Autodesk Inventor part; units mm, degrees
ref_plane "YZ Plane" through (0, 0, 0) normal (1, 0, 0) x (0, 1, 0)
ref_plane "XZ Plane" through (0, 0, 0) normal (0, 1, 0) x (-1, 0, 0)
ref_plane "XY Plane" through (0, 0, 0) normal (0, 0, 1) x (1, 0, 0)
sketch "Sketch1" plane through (0, 0, 0) normal (1, 0, 0) x (0, 1, 0)
  line L0 (15.4505, 45.3153) -> (5.4505, 45.3153)
  line L1 (5.4505, 45.3153) -> (5.4505, 35.3153)
  line L2 (5.4505, 35.3153) -> (15.4505, 35.3153)
  line L3 (15.4505, 35.3153) -> (15.4505, 45.3153)
  line L4 (29.1713, -4.6847) -> (-18.7008, -4.6847)
  point P0 (0, 0)
  dimension "d0" = 10
  dimension "d1" = 10
  dimension "d3" = 100
revolve "Revolution1" add sketch "Sketch1" angle 360 about axis through (0, 29.1713, -4.6847) along (0, -1, 0)
chamfer "Chamfer1" distance 1 angle 45 4 edges at (0, 15.4505, -54.6847) (0, 5.4505, -54.6847) (0, 15.4505, -44.6847) (0, 5.4505, -44.6847)
properties part number "bearing100-80-10" material "Steel, Galvanized"
Geometry check sheet. Reference: the model listing, model coordinates, mm. Round coordinates to 2 decimals unless told otherwise and drop trailing zeros. Write each loop counter-clockwise with the first axis right and the second up, starting at its lowest first coordinate (ties: lowest second). Pieces come first, ordered by that corner, then holes. Notation, with made-up numbers: (86, -38.75) - (113, -38.75) arc R18 cw to (113, -15.75) - close; hole circle Ø6 at (89.25, 20). An arc over 180 degrees is marked (long way). Write each question's results on one line, items separated by ' | '.
(1) Depth check by flat-ended pin: pin 1 Ø1 at (x, z) = (37, -19.5) entering from -Y; pin 2 Ø4 at (x, y) = (12.5, 8.5) entering from -Z; pin 3 Ø2 at (y, z) = (8, -32.5) entering from +X. Enter the tip coordinate at first touch or a pass-through.
Computed:
pin 1: stops at y = 6.09 | pin 2: stops at z = -53.57 | pin 3: stops at x = 42.2
(2) Sectioned sample at B-B, the plane y = 9. Enter the section's corners in (x, z).
Computed:
outline: circle Ø100 at (0, -4.68); hole circle Ø80 at (0, -4.68)
(3) Draft check along Z on faces 1 (the face through (-15.019, 10.394, 43.006)), 2 (the face through (-24.339, 10.506, -36.427)), 3 (the face through (40, 15.45, -16)). Enter one of: pulls with the +Z half, pulls with the -Z half, needs draft (parallel to the pull), parting line crosses it, or undercut.
Computed:
face 1: parting line crosses it | face 2: undercut | face 3: needs draft
(4) Sectioned sample at A-A, the plane x = 0. Enter the section's corners in (y, z).
Computed:
outline: (5.45, -53.68) - (6.45, -54.68) - (14.45, -54.68) - (15.45, -53.68) - (15.45, -45.68) - (14.45, -44.68) - (6.45, -44.68) - (5.45, -45.68) - close; (5.45, 36.32) - (6.45, 35.32) - (14.45, 35.32) - (15.45, 36.32) - (15.45, 44.32) - (14.45, 45.32) - (6.45, 45.32) - (5.45, 44.32) - close
(5) Thickness scan on probe 1 along Z at (x, y) = (0, 10.25); probe 2 along X at (y, z) = (6.5, -28); probe 3 along X at (y, z) = (8, 8). Record the ranges inside material, lowest first. Write a range as from..to.
Computed:
probe 1: z = -54.68..-44.68, 35.32..45.32 | probe 2: x = -44.23..-32.5, 32.5..44.23 | probe 3: x = -48.36..-37.94, 37.94..48.36
